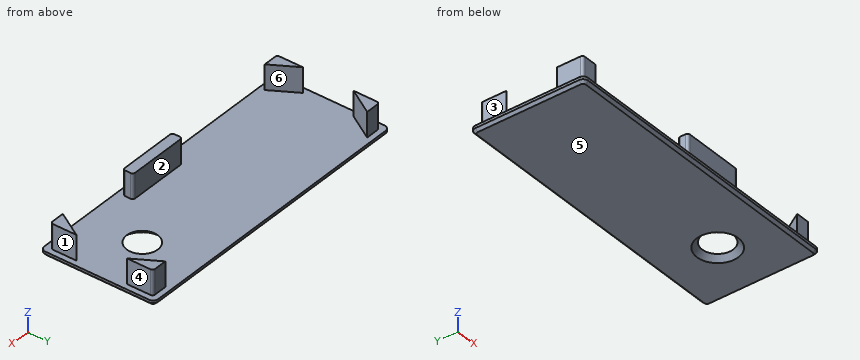
from build123d import *

# Parameters (mm, degrees)
F0_R     = 3
F1_DEPTH = 1
F3_DEPTH = 4.8
F4_SIZE  = 0.99999
F5_SIZE  = 0.5


# Not quite as in the source:
# - a fillet or chamfer is up to 0.001 mm smaller than in the source, because OpenCascade refuses the exact size


with BuildPart() as f1:
    # F0 (on Top) → F1 (new body)
    with BuildSketch(Plane.XY):
        with BuildLine():
            Line((56.5, 22), (1, 22))
            ThreePointArc((1, 22), (0.2928932188, 21.7071067812), (0, 21))
            Line((0, 21), (0, 1))
            ThreePointArc((0, 1), (0.2928932188, 0.2928932188), (1, 0))
            Line((1, 0), (56.5, 0))
            ThreePointArc((56.5, 0), (57.2071067812, 0.2928932188), (57.5, 1))
            Line((57.5, 1), (57.5, 21))
            ThreePointArc((57.5, 21), (57.2071067812, 21.7071067812), (56.5, 22))
        make_face()
        with Locations((46.5, 11)):
            Circle(F0_R, mode=Mode.SUBTRACT)
    extrude(amount=F1_DEPTH)

    # F2 (on face) → F3 (join)
    with BuildSketch(Plane.XY.offset(1)):
        with BuildLine():
            Line((1.1, 20.4), (1.1, 15.9))
            Line((1.1, 15.9), (4.1, 20.9))
            Line((4.1, 20.9), (1.6, 20.9))
            ThreePointArc((1.6, 20.9), (1.2464466094, 20.7535533906), (1.1, 20.4))
        make_face()
        with BuildLine():
            ThreePointArc((56.4, 20.4), (56.2535533906, 20.7535533906), (55.9, 20.9))
            Line((55.9, 20.9), (53.4, 20.9))
            Line((53.4, 20.9), (56.4, 15.9))
            Line((56.4, 15.9), (56.4, 20.4))
        make_face()
        with BuildLine():
            ThreePointArc((1.1, 1.6), (1.2464466094, 1.2464466094), (1.6, 1.1))
            Line((1.6, 1.1), (4.1, 1.1))
            Line((4.1, 1.1), (1.1, 6.1))
            Line((1.1, 6.1), (1.1, 1.6))
        make_face()
        with BuildLine():
            Line((53.4, 1.1), (55.9, 1.1))
            ThreePointArc((55.9, 1.1), (56.2535533906, 1.2464466094), (56.4, 1.6))
            Line((56.4, 1.6), (56.4, 6.1))
            Line((56.4, 6.1), (53.4, 1.1))
        make_face()
        with BuildLine():
            Line((38.25, 3.1), (27.25, 3.1))
            ThreePointArc((27.25, 3.1), (26.8964466094, 2.9535533906), (26.75, 2.6))
            Line((26.75, 2.6), (26.75, 1.6))
            ThreePointArc((26.75, 1.6), (26.8964466094, 1.2464466094), (27.25, 1.1))
            Line((27.25, 1.1), (38.25, 1.1))
            ThreePointArc((38.25, 1.1), (38.6035533906, 1.2464466094), (38.75, 1.6))
            Line((38.75, 1.6), (38.75, 2.6))
            ThreePointArc((38.75, 2.6), (38.6035533906, 2.9535533906), (38.25, 3.1))
        make_face()
    extrude(amount=F3_DEPTH)

    # F4 (size 1 in the source; OpenCascade refuses exactly that, so slightly less here)
    f4_edges = [f1.edges().sort_by_distance(p)[0] for p in [
        (43.5, 11, 0),
    ]]
    chamfer(f4_edges, length=F4_SIZE)

    # F5
    f5_edges = [f1.edges().sort_by_distance(p)[0] for p in [
        (28.75, 0, 0),
        (0, 11, 0),
        (0.292893, 0.292893, 0),
        (0.292893, 21.707107, 0),
        (28.75, 22, 0),
        (57.5, 11, 0),
        (57.207107, 0.292893, 0),
        (57.207107, 21.707107, 0),
    ]]
    chamfer(f5_edges, length=F5_SIZE)


solid = f1.part
Check sheet for the modelled part. Datum: model origin and axes. Units: mm. Face numbers are marked on the shaded views. A direction names the side the tool comes from. Give positions to 0.01 mm unless a question says otherwise; leave off trailing zeros. Order: outer loops, then holes, each group sorted by start corner. A loop starts at its lowest first (then second) coordinate and runs counter-clockwise, first axis right, second up. Notation, with made-up numbers: M 54,-14 L 105,-14 A19 ccw 105,-2 Z; hole C -25.5,54.25 d9. An arc over 180 degrees is marked long. Answer as CSV lines item,"result". Start each with the question number.
Item 1: Gauge pin test, flat ends, axial feed: P1, Ø2.5, axis at x = 3, z = 4.5, coming from the -Y side; P2, Ø3.5, axis at x = 46.5, y = 11, coming from the +Z side; P3, Ø6, axis at x = 20.5, y = 17.5, coming from the +Z side; P4, Ø2, axis at y = 4, z = 4, coming from the +X side. Record the tip position at first contact, or that the pin passes through.
Item 2: Tool access check on the marked faces 1, 2 and 3. Record the directions out of +Z, -Z, +X, -X, +Y, -Y that give a thin tool (end or side, any length) a straight path to the whole face; none if there is none.
Item 3: Thickness scan on line 1 (X direction, y = 2.5, z = 3.85); line 2 (X direction, y = 2.75, z = 3.55); line 3 (Z direction, x = 34.5, y = 6.5). Record the ranges inside material, lowest first. Write a range as [from, to].
Item 4: Mould release check, pull along X, two halves, no side actions. Record for the marked faces 4, 5 and 6: +X half, -X half, draft (parallel to the pull), parting line (faces both ways), or undercut.
Item 5: Cross-section at D-D on y = 19. Enter the section's corners in (x, z).
Item 6: Cross-section at C-C on z = 4.9. Enter the section's corners in (x, y).
Established:
1,P1,"stops at y = 1.1"
1,P2,"passes through"
1,P3,"stops at z = 1"
1,P4,"stops at x = 56.4"
2,face 1,"+Z, +X, +Y, -Y"
2,face 2,"+Z, +Y"
2,face 3,"+Z, -X, +Y, -Y"
3,line 1,"x = [1.1, 3.26], [26.75, 38.75], [54.24, 56.4]"
3,line 2,"x = [1.1, 3.11], [26.77, 38.73], [54.39, 56.4]"
3,line 3,"z = [0, 1]"
4,face 4,"+X half"
4,face 5,"draft"
4,face 6,"undercut"
5,outline,"M 0,0.5 L 0.5,0 L 57,0 L 57.5,0.5 L 57.5,1 L 56.4,1 L 56.4,5.8 L 54.54,5.8 L 54.54,1 L 2.96,1 L 2.96,5.8 L 1.1,5.8 L 1.1,1 L 0,1 Z"
6,outline,"M 1.1,1.6 A0.5 ccw 1.6,1.1 L 4.1,1.1 L 1.1,6.1 Z; M 1.1,15.9 L 4.1,20.9 L 1.6,20.9 A0.5 ccw 1.1,20.4 Z; M 26.75,1.6 A0.5 ccw 27.25,1.1 L 38.25,1.1 A0.5 ccw 38.75,1.6 L 38.75,2.6 A0.5 ccw 38.25,3.1 L 27.25,3.1 A0.5 ccw 26.75,2.6 Z; M 53.4,1.1 L 55.9,1.1 A0.5 ccw 56.4,1.6 L 56.4,6.1 Z; M 53.4,20.9 L 56.4,15.9 L 56.4,20.4 A0.5 ccw 55.9,20.9 Z"
